from build123d import *

# Parameters (mm, degrees)
BOSS_EXTRUDE1_DEPTH = 40
CHAMFER2_SIZE       = 10
CHAMFER2_SIZE2      = 20
SKETCH2_R           = 10
SKETCH2_R_2         = 5
BOSS_EXTRUDE2_DEPTH = 15


with BuildPart() as part:
    # Sketch1 → Boss-Extrude1 (new body)
    with BuildSketch(Plane.YZ):
        Polygon((0, 0), (10, 0), (10, 5), (50, 5), (50, 0), (60, 0), (60, 15), (10, 15), (10, 65), (0, 65), align=None)
    extrude(amount=BOSS_EXTRUDE1_DEPTH)

    # Chamfer2
    chamfer2_edges = [part.edges().sort_by_distance(p)[0] for p in [
        (40, 5, 65),
    ]]
    chamfer2_side = [part.faces().sort_by_distance(p)[0] for p in [
        (20, 5, 65),
    ]]
    chamfer(chamfer2_edges, length=CHAMFER2_SIZE, length2=CHAMFER2_SIZE2, reference=chamfer2_side[0])

    # Sketch2 → Boss-Extrude2 (add)
    with BuildSketch(Plane(origin=(0, 10, 0), x_dir=(-1, 0, 0), z_dir=(0, 1, 0))):
        with Locations(Location((-20, 40, 0), (0, 0, 270))):
            Circle(SKETCH2_R)
        with Locations(Location((-20, 40, 0), (0, 0, 90))):
            Circle(SKETCH2_R_2, mode=Mode.SUBTRACT)
    extrude(amount=BOSS_EXTRUDE2_DEPTH)


solid = part.part
Verification items for the finished model (mm, model axes). A direction names the side the tool comes from. Give positions to 0.01 mm unless a question says otherwise; leave off trailing zeros. Write each loop counter-clockwise with the first axis right and the second up, starting at its lowest first coordinate (ties: lowest second). Pieces come first, ordered by that corner, then holes. Notation, with made-up numbers: M -10.75,-13 L 11.25,-13 A22 cw 11.25,19 Z; hole C 23.5,63.25 d10. An arc over 180 degrees is marked long. Put each result on its own line as item: value. Start each with the question number.
1. Section check B-B (x = 26). Record the cut outline in (y, z).
2. Section check D-D (y = 41). Record the cut outline in (x, z).
3. Go/stop test with flat-tipped pins: pin 1 Ø10 at (x, z) = (16.5, 35) entering from +Y; pin 2 Ø1.5 at (x, z) = (34.5, 37) entering from +Y; pin 3 Ø12 at (x, y) = (24.5, 34) entering from +Z. Record where each tip stops, or that it passes through.
4. Set-up check for faces 1 (the face through (22, 25, 45)), 2 (the face through (20, 0, 33)), 3 (the face through (15, 5, 65)), 4 (the face through (20, 30, 5)), 5 (the face through (11, 10, 34)): record each of +Z, -Z, +X, -X, +Y, -Y from which the full face is reachable in a straight line by a thin tool's end or side.
5. Scan lines: line 1 along X through (y, z) = (13.75, 40); line 2 along Y through (x, z) = (15.5, 21); line 3 along Z through (x, y) = (34, 49). Record each from-to range of solid material in increasing order. Write a range as [from, to].
6. Draft check along X on faces 6 (the face through (17, 17, 36)), 7 (the face through (20, 35, 15)), 8 (the face through (40, 23, 13)). Enter one of: +X half, -X half, draft (parallel to the pull), parting line (faces both ways), or undercut.
7. Section check A-A (y = 12.5). Record the cut outline in (x, z).
8. Section check C-C (z = 40). Record the cut outline in (x, y).
Answer list:
1. outline: M 0,0 L 10,0 L 10,5 L 50,5 L 50,0 L 60,0 L 60,15 L 10,15 L 10,32 L 25,32 L 25,48 L 10,48 L 10,65 L 0,65 Z
2. outline: M 0,5 L 40,5 L 40,15 L 0,15 Z
3. pin 1: y = 25
3. pin 2: y = 10
3. pin 3: z = 15
4. face 1: +Z, +X, -X, +Y
4. face 2: +Z, -Z, +X, -X, -Y
4. face 3: +Z, +X, -X, +Y, -Y
4. face 4: -Z, +X, -X
4. face 5: +Y
5. line 1: [10, 15], [25, 30]
5. line 2: [0, 10]
5. line 3: [5, 15]
6. face 6: undercut
6. face 7: draft
6. face 8: +X half
7. outline: M 0,5 L 40,5 L 40,15 L 0,15 Z; C 20,40 d20; hole C 20,40 d10
8. outline: M 0,0 L 40,0 L 40,10 L 30,10 L 30,25 L 25,25 L 25,10 L 15,10 L 15,25 L 10,25 L 10,10 L 0,10 Z
